```python
from build123d import *

# Parameters (mm, degrees)
SKETCH1_W           = 20
SKETCH1_H           = 32
SKETCH1_R           = 1.1
SKETCH1_W_2         = 12.5
SKETCH1_H_2         = 24
BOSS_EXTRUDE1_DEPTH = 2.5
BOSS_EXTRUDE2_DEPTH = 2.5
CHAMFER1_SIZE       = 11
SKETCH3_R           = 2.2
BOSS_EXTRUDE3_DEPTH = 2.5
SKETCH4_W           = 25
SKETCH4_H           = 32
BOSS_EXTRUDE4_DEPTH = 2.5
SKETCH5_W           = 58
SKETCH5_H           = 32
SKETCH5_R           = 1.2
SKETCH5_W_2         = 42
SKETCH5_H_2         = 21
BOSS_EXTRUDE5_DEPTH = 2.5
CHAMFER2_SIZE       = 2.5


with BuildPart() as part:
    # Sketch1 → Boss-Extrude1 (new body)
    with BuildSketch(Plane(origin=(0, 0, 0), x_dir=(1, 0, 0), z_dir=(0, 1, 0))):
        Rectangle(SKETCH1_W, SKETCH1_H)
        with Locations(Location((0, -13.75, 0), (0, 0, 270))):
            Circle(SKETCH1_R, mode=Mode.SUBTRACT)
        with Locations(Location((0, 13.75, 0), (0, 0, 270))):
            Circle(SKETCH1_R, mode=Mode.SUBTRACT)
        Rectangle(SKETCH1_W_2, SKETCH1_H_2, mode=Mode.SUBTRACT)
    extrude(amount=BOSS_EXTRUDE1_DEPTH)

    # Sketch2 → Boss-Extrude2 (add)
    with BuildSketch(Plane(origin=(0, 2.5, 0), x_dir=(1, 0, 0), z_dir=(0, 1, 0))):
        with BuildLine():
            Line((10, 5), (45, 5))
            ThreePointArc((45, 5), (50, 0), (45, -5))
            Line((45, -5), (10, -5))
            ThreePointArc((10, -5), (7.942810861, -4.557189139), (6.25, -3.307189139))
            Line((6.25, -3.307189139), (6.25, 3.307189139))
            ThreePointArc((6.25, 3.307189139), (7.942810861, 4.557189139), (10, 5))
        make_face()
        with BuildLine():
            Line((10, 2.2), (45, 2.2))
            ThreePointArc((45, 2.2), (47.2, 0), (45, -2.2))
            Line((45, -2.2), (10, -2.2))
            ThreePointArc((10, -2.2), (7.8, 0), (10, 2.2))
        make_face(mode=Mode.SUBTRACT)
    extrude(amount=-BOSS_EXTRUDE2_DEPTH)

    # Chamfer1
    chamfer1_edges = [part.edges().sort_by_distance(p)[0] for p in [
        (10, 1.25, 5),
        (10, 1.25, -5),
    ]]
    chamfer(chamfer1_edges, length=CHAMFER1_SIZE - 0.0001)  # a hair under: the kernel refuses the full size

    # Sketch3 → Boss-Extrude3 (add)
    # profile 1 of 2: a face of its own
    with BuildSketch(Plane(origin=(0, 2.5, 0), x_dir=(1, 0, 0), z_dir=(0, 1, 0))):
        with BuildLine():
            Line((45, -5), (45, -11))
            ThreePointArc((45, -11), (41, -15), (37, -11))
            Line((37, -11), (37, -5))
            Line((37, -5), (45, -5))
        make_face()
        with Locations(Location((41, -11, 0), (0, 0, 270))):
            Circle(SKETCH3_R, mode=Mode.SUBTRACT)
    # profile 2 of 2: a face of its own
    with BuildSketch(Plane(origin=(0, 2.5, 0), x_dir=(1, 0, 0), z_dir=(0, 1, 0))):
        with BuildLine():
            Line((45, 5), (45, 11))
            ThreePointArc((45, 11), (41, 15), (37, 11))
            Line((37, 11), (37, 5))
            Line((37, 5), (45, 5))
        make_face()
        with Locations(Location((41, 11, 0), (0, 0, 90))):
            Circle(SKETCH3_R, mode=Mode.SUBTRACT)
    extrude(amount=-BOSS_EXTRUDE3_DEPTH)

    # Sketch4 → Boss-Extrude4 (add)
    with BuildSketch(Plane(origin=(0, 2.5, 0), x_dir=(1, 0, 0), z_dir=(0, 1, 0))):
        with Locations((-22.5, 0)):
            Rectangle(SKETCH4_W, SKETCH4_H)
    extrude(amount=-BOSS_EXTRUDE4_DEPTH)

    # Sketch5 → Boss-Extrude5 (add)
    with BuildSketch(Plane.ZY.offset(35)):
        with Locations((0, -16)):
            Rectangle(SKETCH5_W, SKETCH5_H)
        with Locations((25, -10.5)):
            Circle(SKETCH5_R, mode=Mode.SUBTRACT)
        with Locations((25, -21.5)):
            Circle(SKETCH5_R, mode=Mode.SUBTRACT)
        with Locations((-25, -10.5)):
            Circle(SKETCH5_R, mode=Mode.SUBTRACT)
        with Locations((-25, -21.5)):
            Circle(SKETCH5_R, mode=Mode.SUBTRACT)
        with Locations((0, -16)):
            Rectangle(SKETCH5_W_2, SKETCH5_H_2, mode=Mode.SUBTRACT)
    extrude(amount=-BOSS_EXTRUDE5_DEPTH)

    # Chamfer2
    chamfer2_edges = [part.edges().sort_by_distance(p)[0] for p in [
        (-33.75, 0, -16),
        (-33.75, 0, 16),
    ]]
    chamfer(chamfer2_edges, length=CHAMFER2_SIZE - 0.0001)  # a hair under: the kernel refuses the full size


solid = part.part
```
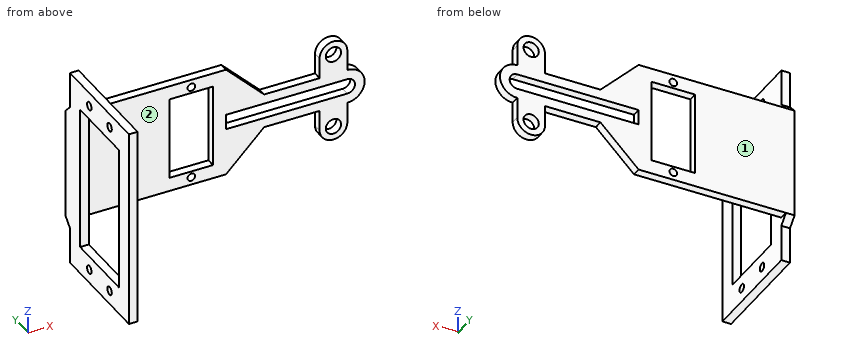
Here's how the part is built. I have some questions about the finished solid (model axes, mm). Face numbers are marked on the shaded views. A direction names the side the tool comes from. Give positions to 0.01 mm unless a question says otherwise; leave off trailing zeros. Loops run counter-clockwise (first coordinate to the right, second up) from the corner with the lowest first, then second, coordinate; pieces in that order, holes last. Notation, with made-up numbers: M 81,79.25 L 131,79.25 A16 ccw 131,105.25 Z; hole C 75,-27 d2. An arc over 180 degrees is marked long. Put each result on its own line as item: value. Start each with the question number.
(1) I want a section at B-B on y = -14. Please give me the cut outline in (x, z), then the cut area to 3 significant figures.
(2) I need wall thicknesses on line 1 along X through (y, z) = (0.9, -11); line 2 along Y through (x, z) = (-32.95, 25); line 3 along X through (y, z) = (1.9, -13.75). Which ranges of each line are inside material? Lowest first, please. Write a range as [from, to].
(3) Will these pins go through, and if not, where does the flat tip stop? pin 1 Ø16 at (x, z) = (18.5, 0.5) entering from -Y; pin 2 Ø1.2 at (x, y) = (26, 1.5) entering from +Z; pin 3 Ø8 at (y, z) = (-14, 20.5) entering from -X; pin 4 Ø2 at (x, z) = (-33.5, -23.5) entering from +Y.
(4) I want a section at A-A on x = 24. Please give me the cut outline in (y, z), then the cut area to 3 significant figures.
(5) For the marked faces 1 and 2, which set-ups out of +Z, -Z, +X, -X, +Y, -Y let a thin tool reach every point of the face, with its end or its side?
(6) I want a section at D-D on x = 0. Please give me the cut outline in (y, z), then the cut area to 3 significant figures.
(7) I want a section at C-C on z = -25. Please give me the cut outline in (x, y), then the cut area to 3 significant figures.
Answer block:
1. outline: M -35,-29 L -32.5,-29 L -32.5,-21 L -35,-21 Z; M -35,21 L -32.5,21 L -32.5,29 L -35,29 Z
1. area: 40.0 mm^2
2. line 1: [-35, -6.25], [6.25, 15], [37, 38.8], [43.2, 45]
2. line 2: [-32, -22.7], [-20.3, -11.7], [-9.3, 0]
2. line 3: [-35, -1.1], [1.1, 12.25], [38.1, 43.9]
3. pin 1: y = 0
3. pin 2: z = 5
3. pin 3: x = -35
3. pin 4: y = 0
4. outline: M 0,-5 L 2.5,-5 L 2.5,-2.2 L 0,-2.2 Z; M 0,2.2 L 2.5,2.2 L 2.5,5 L 0,5 Z
4. area: 14.0 mm^2
5. face 1: +Z, -Z, +X, -X, +Y
5. face 2: +Z, -Z, +X, -Y
6. outline: M 0,-16 L 2.5,-16 L 2.5,-14.85 L 0,-14.85 Z; M 0,-12.65 L 2.5,-12.65 L 2.5,-12 L 0,-12 Z; M 0,12 L 2.5,12 L 2.5,12.65 L 0,12.65 Z; M 0,14.85 L 2.5,14.85 L 2.5,16 L 0,16 Z
6. area: 9.00 mm^2
7. outline: M -35,-32 L -32.5,-32 L -32.5,-22.7 L -35,-22.7 Z; M -35,-20.3 L -32.5,-20.3 L -32.5,-11.7 L -35,-11.7 Z; M -35,-9.3 L -32.5,-9.3 L -32.5,0 L -35,0 Z
7. area: 68.0 mm^2
